from build123d import *

# Parameters (mm, degrees)
F1_DEPTH  = 152.4
F2_DEPTH  = 12.7
F3_DEPTH  = 76.2
F4_W      = 12.7
F4_H      = 227.33
F5_DEPTH  = 25.4
F6_DEPTH  = 133.35
F8_DEPTH  = 12.7
F10_DEPTH = 12.7


with BuildPart() as f1:
    # F0 (on Front) → F1 (new body, symmetric)
    with BuildSketch(Plane.XZ):
        Polygon((231.775, -973.5972180367), (-231.775, -973.5972180367), (-244.475, -973.5972180367), (-244.475, -992.6472180367), (244.475, -992.6472180367), (244.475, -973.5972180367), align=None)
    extrude(amount=F1_DEPTH, both=True)

    # F0 (on Front) → F2 (join)
    with BuildSketch(Plane.XZ):
        with BuildLine():
            ThreePointArc((260.0142581205, -699.6271664014), (0, -751.3472180367), (-260.0142581205, -699.6271664014))
            Line((-260.0142581205, -699.6271664014), (-264.8743377115, -711.3604364643))
            ThreePointArc((-264.8743377115, -711.3604364643), (-259.0018869142, -713.7614132329), (-253.1076754433, -716.1084622195))
            ThreePointArc((-253.1076754433, -716.1084622195), (0.5785166895, -764.0469762671), (254.1842179232, -715.6844545199))
            ThreePointArc((254.1842179232, -715.6844545199), (259.5382829708, -713.5447086205), (264.8743377115, -711.3604364643))
            Line((264.8743377115, -711.3604364643), (260.0142581205, -699.6271664014))
        make_face()
        with BuildLine():
            ThreePointArc((254.1842179232, -715.6844545199), (0.5785166895, -764.0469762671), (-253.1076754433, -716.1084622195))
            Line((-253.1076754433, -716.1084622195), (-231.775, -973.5972180367))
            Line((-231.775, -973.5972180367), (231.775, -973.5972180367))
            Line((231.775, -973.5972180367), (254.1842179232, -715.6844545199))
        make_face()
        Polygon((231.775, -973.5972180367), (-231.775, -973.5972180367), (-244.475, -973.5972180367), (-244.475, -992.6472180367), (244.475, -992.6472180367), (244.475, -973.5972180367), align=None)
    extrude(amount=F2_DEPTH)

    # F0 (on Front) → F3 (join, symmetric)
    with BuildSketch(Plane.XZ):
        with BuildLine():
            ThreePointArc((260.0142581205, -699.6271664014), (0, -751.3472180367), (-260.0142581205, -699.6271664014))
            Line((-260.0142581205, -699.6271664014), (-264.8743377115, -711.3604364643))
            ThreePointArc((-264.8743377115, -711.3604364643), (-259.0018869142, -713.7614132329), (-253.1076754433, -716.1084622195))
            ThreePointArc((-253.1076754433, -716.1084622195), (0.5785166895, -764.0469762671), (254.1842179232, -715.6844545199))
            ThreePointArc((254.1842179232, -715.6844545199), (259.5382829708, -713.5447086205), (264.8743377115, -711.3604364643))
            Line((264.8743377115, -711.3604364643), (260.0142581205, -699.6271664014))
        make_face()
    extrude(amount=F3_DEPTH, both=True)

    # F4 (on face) → F5 (join)
    with BuildSketch(Plane.XZ.offset(12.7)):
        with Locations((-169.8625, -859.9322180367)):
            Rectangle(F4_W, F4_H)
        with Locations((169.8625, -859.9322180367)):
            Rectangle(F4_W, F4_H)
    extrude(amount=F5_DEPTH)

    # F4 (on face) → F6 (join)
    with BuildSketch(Plane.XZ.offset(12.7)):
        with Locations((-169.8625, -859.9322180367)):
            Rectangle(F4_W, F4_H)
        with Locations((169.8625, -859.9322180367)):
            Rectangle(F4_W, F4_H)
    extrude(amount=F6_DEPTH)

    # F7 (on face) → F8 (cut)
    with BuildSketch(Plane(origin=(-176.2125, 0, 0), x_dir=(0, -1, 0), z_dir=(-1, 0, 0))):
        Polygon((146.05, -746.2672180367), (69.85, -746.2672180367), (146.05, -973.5972180367), align=None)
    extrude(amount=-F8_DEPTH, mode=Mode.SUBTRACT)

    # F9 (on face) → F10 (cut)
    with BuildSketch(Plane.YZ.offset(176.2125)):
        Polygon((-146.05, -973.5972180367), (-69.85, -746.2672180367), (-146.05, -746.2672180367), align=None)
    extrude(amount=-F10_DEPTH, mode=Mode.SUBTRACT)


solid = f1.part
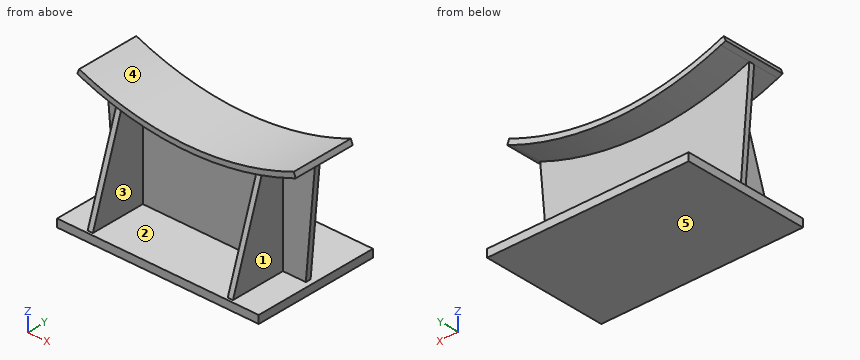
CAD build for the part. Positions are in the model's coordinates, mm. Face numbers are marked on the shaded views. A direction names the side the tool comes from. Coordinates: 2 decimals unless noted, no trailing zeros. Order: outer loops, then holes, each group sorted by start corner. A loop starts at its lowest first (then second) coordinate and runs counter-clockwise, first axis right, second up. Notation, with made-up numbers: (62, 26) -> (119, 26) arc R14 cw to (119, 37) -> close; hole circle Ø7 at (33.25, -32). An arc over 180 degrees is marked (long way). Answer in a Markdown table with one row per item.
1) Mould opens along Z. For the marked faces 3, 4 and 5 say: pulls with the +Z half, pulls with the -Z half, needs draft (parallel to the pull), parting line crosses it, or undercut.
Check values:
| item | result |
|---|---|
| face 3 | undercut |
| face 4 | pulls with the +Z half |
| face 5 | pulls with the -Z half |
2) Which spindle directions (+Z, -Z, +X, -X, +Y, -Y) get a long thin tool onto all of the face, cutting with end or side? Do the marked faces 1 and 2. Say none if no direction does.
Check values:
| item | result |
|---|---|
| face 1 | +X, -Y |
| face 2 | none |
3) Flat gauge pins, fed straight in: P1, Ø9.5, axis at y = 7, z = -987.5, coming from the +X side (3 decimals); P2, Ø10, axis at x = 169, y = -31.5, coming from the +Z side; P3, Ø6, axis at x = -125.5, z = -879, coming from the -Y side. Where does each tip first touch, or does it go through?
Check values:
| item | result |
|---|---|
| P1 | x = 244.475 |
| P2 | z = -728.69 |
| P3 | y = -12.7 |
4) Drill centre lines: line 1 (Z direction, x = 5.5, y = 60.5); line 2 (X direction, y = -44, z = -781.5); line 3 (Y direction, x = 237.5, z = -838). Where is each one in solid material? Low to high.
Check values:
| item | result |
|---|---|
| line 1 | -992.65 to -973.6, -764.03 to -751.32 |
| line 2 | -176.21 to -163.51, 163.51 to 176.21 |
| line 3 | -12.7 to 0 |
5) Band-saw the part on A-A (y = 17). List the corners of the cut face in (x, z) (3 decimals), and give its area (3 significant figures).
Check values:
| item | result |
|---|---|
| outline | (-264.874, -711.36) arc R692.15 ccw to (-253.108, -716.108) arc R692.15 ccw to (264.874, -711.36) -> (260.014, -699.627) arc R679.45 cw to (-260.014, -699.627) -> close; (-244.475, -992.647) -> (244.475, -992.647) -> (244.475, -973.597) -> (-244.475, -973.597) -> close |
| area | 16,200 mm2 |
6) Band-saw the part on B-B (z = -732.5). List the corners of the cut face in (x, y).
Check values:
| item | result |
|---|---|
| outline | (-251.75, -12.7) -> (-206.58, -12.7) -> (-206.58, -76.2) -> (-158.92, -76.2) -> (-158.92, 76.2) -> (-206.58, 76.2) -> (-206.58, 0) -> (-251.75, 0) -> close; (158.92, -76.2) -> (206.58, -76.2) -> (206.58, -12.7) -> (252.72, -12.7) -> (252.72, 0) -> (206.58, 0) -> (206.58, 76.2) -> (158.92, 76.2) -> close |
7) Band-saw the part on D-D (z = -780). List the corners of the cut face in (x, y).
Check values:
| item | result |
|---|---|
| outline | (-247.81, -12.7) -> (-176.21, -12.7) -> (-176.21, -81.16) -> (-163.51, -81.16) -> (-163.51, -12.7) -> (163.51, -12.7) -> (163.51, -81.16) -> (176.21, -81.16) -> (176.21, -12.7) -> (248.6, -12.7) -> (248.6, 0) -> (-247.81, 0) -> close |
8) Band-saw the part on C-C (x = -122). List the corners of the cut face in (y, z).
Check values:
| item | result |
|---|---|
| outline | (-152.4, -992.65) -> (152.4, -992.65) -> (152.4, -973.6) -> (0, -973.6) -> (0, -753.21) -> (76.2, -753.21) -> (76.2, -740.3) -> (-76.2, -740.3) -> (-76.2, -753.21) -> (-12.7, -753.21) -> (-12.7, -973.6) -> (-152.4, -973.6) -> close |
